Geometry check sheet. Reference: the model listing, model coordinates, mm. Face numbers are marked on the shaded views. Round coordinates to 2 decimals unless told otherwise and drop trailing zeros. Loops run counter-clockwise (first coordinate to the right, second up) from the corner with the lowest first, then second, coordinate; pieces in that order, holes last.
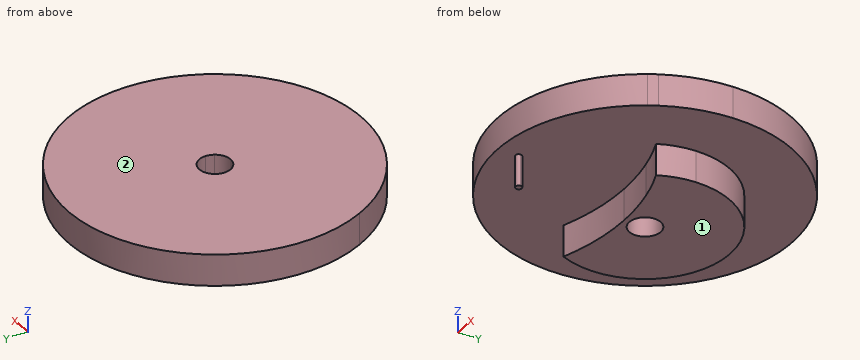
```python
from build123d import *

# Parameters (mm, degrees)
F1_DEPTH = 12.7
F2_DEPTH = 12.7


with BuildPart() as f1:
    # F0 (on Top) → F1 (new body)
    with BuildSketch(Plane.XY):
        with BuildLine():
            Line((1.27, 0), (0, 0))
            Line((0, 0), (0, 1.27))
            ThreePointArc((0, 1.27), (-0.8980256121, -0.8980256121), (1.27, 0))
        make_face()
        with BuildLine():
            Line((0, 1.27), (0, 0))
            Line((0, 0), (1.27, 0))
            ThreePointArc((1.27, 0), (0.8980256121, 0.8980256121), (0, 1.27))
        make_face()
        with BuildLine():
            ThreePointArc((1.27, 0), (-0.8980256121, -0.8980256121), (0, 1.27))
            Line((0, 1.27), (0, 16.51))
            ThreePointArc((0, 16.51), (-18.5637162853, 21.9695900536), (-31.2160717781, 36.6098286569))
            ThreePointArc((-31.2160717781, 36.6098286569), (-42.6516552572, 31.3045995485), (-53.2117304222, 24.4196276597))
            ThreePointArc((-53.2117304222, 24.4196276597), (-16.5828563916, -6.2300023956), (30.7696652459, 0))
            Line((30.7696652459, 0), (1.27, 0))
        make_face()
        with BuildLine():
            Line((0, 16.51), (0, 1.27))
            ThreePointArc((0, 1.27), (0.8980256121, 0.8980256121), (1.27, 0))
            Line((1.27, 0), (30.7696652459, 0))
            ThreePointArc((30.7696652459, 0), (42.4352015878, 9.2468296571), (51.4349999952, 21.103988907))
            Line((51.4349999952, 21.103988907), (29.6960110958, 33.655))
            ThreePointArc((29.6960110958, 33.655), (17.145, 21.1039889042), (0, 16.51))
        make_face()
        with BuildLine():
            ThreePointArc((-31.2160717781, 36.6098286569), (-18.5637162853, 21.9695900536), (0, 16.51))
            Line((0, 16.51), (0, 42.3333333333))
            ThreePointArc((0, 42.3333333333), (-15.8682201509, 40.8906294723), (-31.2160717781, 36.6098286569))
        make_face()
        with BuildLine():
            Line((0, 42.3333333333), (0, 16.51))
            ThreePointArc((0, 16.51), (17.145, 21.1039889042), (29.6960110958, 33.655))
            Line((29.6960110958, 33.655), (17.8245764663, 40.508975979))
            ThreePointArc((17.8245764663, 40.508975979), (8.9588476653, 41.8760557513), (0, 42.3333333333))
        make_face()
        with BuildLine():
            ThreePointArc((-31.2160717781, 36.6098286569), (-15.8682201509, 40.8906294723), (0, 42.3333333333))
            Line((0, 42.3333333333), (0, 44.45))
            ThreePointArc((0, 44.45), (-4.4901280605, 55.2901280605), (6.35, 50.8))
            ThreePointArc((6.35, 50.8), (6.1336289969, 49.1564990636), (5.499261314, 47.625))
            Line((5.499261314, 47.625), (17.8245764663, 40.508975979))
            ThreePointArc((17.8245764663, 40.508975979), (24.5977058385, 38.8251673187), (31.2160717781, 36.6098286569))
            ThreePointArc((31.2160717781, 36.6098286569), (33.5127080469, 43.5403512919), (34.29, 50.8))
            ThreePointArc((34.29, 50.8), (-7.2596487081, 84.3127080469), (-31.2160717781, 36.6098286569))
        make_face()
        with BuildLine():
            Line((0, 44.45), (0, 42.3333333333))
            ThreePointArc((0, 42.3333333333), (8.9588476653, 41.8760557513), (17.8245764663, 40.508975979))
            Line((17.8245764663, 40.508975979), (5.499261314, 47.625))
            ThreePointArc((5.499261314, 47.625), (3.175, 45.300738686), (0, 44.45))
        make_face()
        with BuildLine():
            ThreePointArc((-53.2117304222, 24.4196276597), (-42.6516552572, 31.3045995485), (-31.2160717781, 36.6098286569))
            ThreePointArc((-31.2160717781, 36.6098286569), (-7.2596487081, 84.3127080469), (34.29, 50.8))
            ThreePointArc((34.29, 50.8), (33.5127080469, 43.5403512919), (31.2160717781, 36.6098286569))
            ThreePointArc((31.2160717781, 36.6098286569), (42.6516552572, 31.3045995485), (53.2117304222, 24.4196276597))
            ThreePointArc((53.2117304222, 24.4196276597), (57.8263113692, 37.2526750694), (59.392022186, 50.8))
            ThreePointArc((59.392022186, 50.8), (-13.5473249306, 108.6263113692), (-53.2117304222, 24.4196276597))
        make_face()
        with BuildLine():
            ThreePointArc((31.2160717781, 36.6098286569), (30.4918548649, 35.1139907276), (29.6960110958, 33.655))
            Line((29.6960110958, 33.655), (51.4349999952, 21.103988907))
            ThreePointArc((51.4349999952, 21.103988907), (52.3496218883, 22.7477382821), (53.2117304222, 24.4196276597))
            ThreePointArc((53.2117304222, 24.4196276597), (42.6516552572, 31.3045995485), (31.2160717781, 36.6098286569))
        make_face()
        with BuildLine():
            Line((17.8245764663, 40.508975979), (29.6960110958, 33.655))
            ThreePointArc((29.6960110958, 33.655), (30.4918548649, 35.1139907276), (31.2160717781, 36.6098286569))
            ThreePointArc((31.2160717781, 36.6098286569), (24.5977058385, 38.8251673187), (17.8245764663, 40.508975979))
        make_face()
    extrude(amount=F1_DEPTH)

    # F0 (on Top) → F2 (join)
    with BuildSketch(Plane.XY):
        with BuildLine():
            Line((0, 1.27), (0, 0))
            Line((0, 0), (1.27, 0))
            ThreePointArc((1.27, 0), (0.8980256121, 0.8980256121), (0, 1.27))
        make_face()
        with BuildLine():
            Line((1.27, 0), (0, 0))
            Line((0, 0), (0, 1.27))
            ThreePointArc((0, 1.27), (-0.8980256121, -0.8980256121), (1.27, 0))
        make_face()
        with BuildLine():
            ThreePointArc((-31.2160717781, 36.6098286569), (-15.8682201509, 40.8906294723), (0, 42.3333333333))
            Line((0, 42.3333333333), (0, 44.45))
            ThreePointArc((0, 44.45), (-4.4901280605, 55.2901280605), (6.35, 50.8))
            ThreePointArc((6.35, 50.8), (6.1336289969, 49.1564990636), (5.499261314, 47.625))
            Line((5.499261314, 47.625), (17.8245764663, 40.508975979))
            ThreePointArc((17.8245764663, 40.508975979), (24.5977058385, 38.8251673187), (31.2160717781, 36.6098286569))
            ThreePointArc((31.2160717781, 36.6098286569), (33.5127080469, 43.5403512919), (34.29, 50.8))
            ThreePointArc((34.29, 50.8), (-7.2596487081, 84.3127080469), (-31.2160717781, 36.6098286569))
        make_face()
        with BuildLine():
            Line((0, 44.45), (0, 42.3333333333))
            ThreePointArc((0, 42.3333333333), (8.9588476653, 41.8760557513), (17.8245764663, 40.508975979))
            Line((17.8245764663, 40.508975979), (5.499261314, 47.625))
            ThreePointArc((5.499261314, 47.625), (3.175, 45.300738686), (0, 44.45))
        make_face()
    extrude(amount=-F2_DEPTH)


solid = f1.part
```
1) Gauge pin test, flat ends, axial feed: pin 1 (6 mm diameter, centred on y = 96.5, z = 8.5, fed in from +X); pin 2 (6 mm diameter, centred on y = 74.5, z = 6, fed in from +X); pin 3 (1 mm diameter, centred on x = -22.5, y = 4.5, fed in from -Z). Record the tip position at first contact, or that the pin passes through.
Report:
pin 1: stops at x = 41.28
pin 2: stops at x = 55.67
pin 3: stops at z = 0
2) Mould release check, pull along Z, two halves, no side actions. Record for the marked faces 1 and 2: +Z half, -Z half, draft (parallel to the pull), parting line (faces both ways), or undercut.
Report:
face 1: -Z half
face 2: +Z half
3) Sectioned sample at D-D, the plane y = 66.5. Record the cut outline in (x, z).
Report:
outline: (-57.28, 0) - (-30.48, 0) - (-30.48, -12.7) - (30.48, -12.7) - (30.48, 0) - (57.28, 0) - (57.28, 12.7) - (-57.28, 12.7) - close
4) Sectioned sample at A-A, the plane z = -7.5. Record the cut outline in (x, y) (3 decimals), then the cut area to 3 significant figures.
Report:
outline: (-31.216, 36.61) arc R87.988 cw to (31.216, 36.61) arc R34.29 ccw (long way) to start; circle Ø2.54 at (0, 0); hole circle Ø12.7 at (0, 50.8)
area: 2,430 mm2
5) Sectioned sample at B-B, the plane y = 52.5. Record the cut outline in (x, z).
Report:
outline: (-59.37, 0) - (-34.25, 0) - (-34.25, -12.7) - (-6.12, -12.7) - (-6.12, 12.7) - (-59.37, 12.7) - close; (6.12, -12.7) - (34.25, -12.7) - (34.25, 0) - (59.37, 0) - (59.37, 12.7) - (6.12, 12.7) - close
6) Sectioned sample at C-C, the plane x = 4. Record the cut outline in (y, z), then the cut area to 3 significant figures.
Report:
outline: (-8.46, 0) - (42.24, 0) - (42.24, -12.7) - (45.87, -12.7) - (45.87, 12.7) - (-8.46, 12.7) - close; (55.73, -12.7) - (84.86, -12.7) - (84.86, 0) - (110.06, 0) - (110.06, 12.7) - (55.73, 12.7) - close
area: 1,800 mm2
7) Scan lines: line 1 along X through (y, z) = (50.8, 9); line 2 along X through (y, z) = (50.8, -7); line 3 along Z through (x, y) = (42.5, 68). Record each from-to range of solid material in increasing order.
Report:
line 1: x = -59.39 to -6.35, 6.35 to 59.39
line 2: x = -34.29 to -6.35, 6.35 to 34.29
line 3: z = 0 to 12.7
